```python
from build123d import *

# Parameters (mm, degrees)
SKETCH1_W           = 25
SKETCH1_H           = 60
BOSS_EXTRUDE1_DEPTH = 30
SKETCH2_W           = 60
SKETCH2_H           = 8.623813306
BOSS_EXTRUDE2_DEPTH = 20
SKETCH3_R           = 4
CUT_EXTRUDE1_DEPTH  = 9.623813306
CUT_EXTRUDE2_DEPTH  = 20
BOSS_EXTRUDE3_DEPTH = 1


with BuildPart() as part:
    # Sketch1 → Boss-Extrude1 (new body)
    with BuildSketch(Plane(origin=(0, 0, 0), x_dir=(1, 0, 0), z_dir=(0, 1, 0))):
        Rectangle(SKETCH1_W, SKETCH1_H)
    extrude(amount=BOSS_EXTRUDE1_DEPTH)

    # Sketch2 → Boss-Extrude2 (add)
    with BuildSketch(Plane.ZY.offset(12.5)):
        with Locations((0, 4.311906653)):
            Rectangle(SKETCH2_W, SKETCH2_H)
    extrude(amount=BOSS_EXTRUDE2_DEPTH)

    # Sketch3 → Cut-Extrude1 (cut, through all)
    with BuildSketch(Plane(origin=(0, 8.623813306, 0), x_dir=(1, 0, 0), z_dir=(0, 1, 0))):
        with Locations(Location((-24.5, 20, 0), (0, 0, 270))):  # turned: the seam where the file's is
            Circle(SKETCH3_R)
        with Locations(Location((-24.5, -20, 0), (0, 0, 270))):  # turned: the seam where the file's is
            Circle(SKETCH3_R)
    extrude(amount=-CUT_EXTRUDE1_DEPTH, mode=Mode.SUBTRACT)

    # Sketch4 → Cut-Extrude2 (cut)
    with BuildSketch(Plane(origin=(12.5, 0, 0), x_dir=(0, 0, -1), z_dir=(1, 0, 0))):
        Polygon((12.414671802, 26.015265685), (25.398981518, 10.541167934), (17.585328198, 3.984734315), (4.601018482, 19.458832066), align=None)
    extrude(amount=-CUT_EXTRUDE2_DEPTH, mode=Mode.SUBTRACT)

    # Sketch5 → Boss-Extrude3 (add)
    with BuildSketch(Plane(origin=(0, 30, 0), x_dir=(1, 0, 0), z_dir=(0, 1, 0))):
        with BuildLine():
            Line((7.692307692, 10), (7.692307692, -10))
            Line((7.692307692, -10), (-0.985576923, -10))
            add(Edge.make_bspline(
                [(-0.985576923, -10), (-1.189915508, -9.998406517), (-1.585388921, -9.995322517), (-2.158891161, -9.97328499), (-2.692933181, -9.926466249), (-3.190880742, -9.87417544), (-3.651881782, -9.796967041), (-4.076156001, -9.706387661), (-4.462076213, -9.599333368), (-4.812578849, -9.472790754), (-5.13779529, -9.329673653), (-5.439160579, -9.1529927), (-5.729614752, -8.959721513), (-5.997579665, -8.730765608), (-6.255124362, -8.484777239), (-6.491466209, -8.20944831), (-6.713599726, -7.911670049), (-6.98368474, -7.480457665), (-7.26734754, -6.902448182), (-7.511671117, -6.168093018), (-7.667028651, -5.399134972), (-7.683798939, -4.873873893), (-7.692307692, -4.607371795)],
                knots=[0, 0, 0, 0, 1.242075696, 2.40389213, 3.487198984, 4.500157661, 5.446319301, 6.326791195, 7.136300648, 7.878370406, 8.590488565, 9.292260633, 9.999224673, 10.708050372, 11.431369221, 12.162165018, 12.910600795, 13.687589445, 15.252257874, 16.810406251, 18.381693487, 20, 20, 20, 20], degree=3))
            add(Edge.make_bspline(
                [(-7.692307692, -4.607371795), (-7.688394011, -4.436288612), (-7.680664221, -4.098387595), (-7.621454116, -3.601582104), (-7.51431592, -3.126906532), (-7.376939813, -2.670193942), (-7.1888858, -2.237951011), (-6.971132957, -1.821215885), (-6.700987613, -1.431932834), (-6.399355855, -1.057091635), (-6.048612719, -0.71360816), (-5.658467411, -0.39614679), (-5.217190586, -0.123711561), (-4.739255324, 0.129469087), (-4.212344466, 0.337396306), (-3.644404331, 0.520482963), (-3.031039376, 0.661647942), (-2.605906991, 0.732754289), (-2.387820513, 0.769230769)],
                knots=[0, 0, 0, 0, 0.982645791, 1.940792824, 2.867691729, 3.775150443, 4.675643875, 5.571354211, 6.471357401, 7.392684514, 8.331098131, 9.285922955, 10.275520706, 11.304845665, 12.388884831, 13.524255008, 14.729980297, 16, 16, 16, 16], degree=3))
            add(Edge.make_bspline(
                [(-2.387820513, 0.769230769), (-2.549345996, 0.849743746), (-2.855664626, 1.002429402), (-3.272498706, 1.255059029), (-3.637663897, 1.492888205), (-3.845092801, 1.671226556), (-3.942307692, 1.754807692)],
                knots=[0, 0, 0, 0, 1.172551213, 2.223638478, 3.167479604, 4, 4, 4, 4], degree=3))
            add(Edge.make_bspline(
                [(-3.942307692, 1.754807692), (-4.131560958, 1.939760877), (-4.519688241, 2.319069404), (-5.049338611, 2.971134565), (-5.573421338, 3.688219618), (-5.888069662, 4.2107727), (-6.049679487, 4.479166667)],
                knots=[0, 0, 0, 0, 0.918170575, 1.883016652, 2.912673989, 4, 4, 4, 4], degree=3))
            Line((-6.049679487, 4.479166667), (-9.330929487, 10))
            Line((-9.330929487, 10), (-6.09775641, 10))
            Line((-6.09775641, 10), (-3.605769231, 5.77724359))
            add(Edge.make_bspline(
                [(-3.605769231, 5.77724359), (-3.516164402, 5.629086783), (-3.342524957, 5.34198322), (-3.091798881, 4.922621923), (-2.845639404, 4.536751784), (-2.618440056, 4.172360633), (-2.395792195, 3.839058208), (-2.196203285, 3.524230537), (-1.99576396, 3.245712753), (-1.765615132, 2.91110533), (-1.484546035, 2.549334189), (-1.156558274, 2.177690005), (-0.854995349, 1.869836465), (-0.473923576, 1.576103263), (-8.0808e-05, 1.307161834), (0.399436219, 1.179583217), (0.592948718, 1.117788462)],
                knots=[0, 0, 0, 0, 1.130591283, 2.190900266, 3.190104209, 4.119071823, 4.994606968, 5.807262858, 6.55236009, 7.234593472, 8.459046683, 9.540234366, 10.471327768, 11.266723835, 12.676093724, 14, 14, 14, 14], degree=3))
            add(Edge.make_bspline(
                [(0.592948718, 1.117788462), (0.674242958, 1.103128347), (0.859840146, 1.069658866), (1.174983707, 1.047799895), (1.556818794, 1.024599522), (1.833541189, 1.025275503), (1.983173077, 1.025641026)],
                knots=[0, 0, 0, 0, 0.709978628, 1.620902492, 2.713552433, 4, 4, 4, 4], degree=3))
            Line((1.983173077, 1.025641026), (4.871794872, 1.025641026))
            Line((4.871794872, 1.025641026), (4.871794872, 10))
            Line((4.871794872, 10), (7.692307692, 10))
        make_face()
        with BuildLine():
            Line((4.871794872, -1.282051282), (-0.484775641, -1.282051282))
            add(Edge.make_bspline(
                [(-0.484775641, -1.282051282), (-0.753386517, -1.286217416), (-1.255529355, -1.294005613), (-1.957518176, -1.361528247), (-2.558000395, -1.467075801), (-3.064646298, -1.627384754), (-3.490432782, -1.842070076), (-3.859462924, -2.104609449), (-4.169752828, -2.430321342), (-4.424939479, -2.80379836), (-4.624425797, -3.210810832), (-4.763816724, -3.641583566), (-4.857398907, -4.087856282), (-4.866967535, -4.393220511), (-4.871794872, -4.547275641)],
                knots=[0, 0, 0, 0, 1.546056516, 2.890207646, 4.055830773, 5.050253158, 5.937355789, 6.790906573, 7.644595853, 8.512568064, 9.38593768, 10.244184789, 11.114197691, 12, 12, 12, 12], degree=3))
            add(Edge.make_bspline(
                [(-4.871794872, -4.547275641), (-4.868088958, -4.659544766), (-4.86083016, -4.879447), (-4.822372143, -5.202097101), (-4.749202425, -5.50786025), (-4.648165007, -5.798940542), (-4.520236894, -6.075969951), (-4.363033481, -6.337858904), (-4.177365929, -6.583269781), (-3.964383478, -6.81341075), (-3.719926868, -7.02284832), (-3.440676061, -7.203538998), (-3.128860999, -7.357089463), (-2.784111469, -7.478956731), (-2.407515729, -7.576430897), (-1.996929252, -7.641277267), (-1.554229928, -7.688199899), (-1.24746496, -7.690912847), (-1.08974359, -7.692307692)],
                knots=[0, 0, 0, 0, 0.965235723, 1.89061323, 2.787065514, 3.661873922, 4.534873316, 5.404925039, 6.281839248, 7.175200054, 8.095223355, 9.040740021, 10.02630299, 11.075573487, 12.177989335, 13.364883635, 14.645170704, 16, 16, 16, 16], degree=3))
            Line((-1.08974359, -7.692307692), (4.871794872, -7.692307692))
            Line((4.871794872, -7.692307692), (4.871794872, -1.282051282))
        make_face(mode=Mode.SUBTRACT)
    extrude(amount=BOSS_EXTRUDE3_DEPTH)


solid = part.part
```
For this review, take the finished solid that the model builds, in its own axes (mm). A direction names the side the tool comes from. Round coordinates to 2 decimals unless told otherwise and drop trailing zeros. Write each loop counter-clockwise with the first axis right and the second up, starting at its lowest first coordinate (ties: lowest second). Pieces come first, ordered by that corner, then holes. Notation, with made-up numbers: M -8.5,-37 L -3.5,-37 A22 ccw -3.5,-4 Z; hole C 46.25,82.25 d10. An arc over 180 degrees is marked long. One line per item, written item: value. Start each with the question number.
(1) We need section D-D (z = 11). Give the boundary of the cut face in (x, y), and give its area (3 significant figures).
(2) We need section A-A (z = 20). Give the boundary of the cut face in (x, y).
(3) We need section C-C (x = 3). Give the boundary of the cut face in (y, z).
(4) Insertion check: pin 1 (0.8 mm diameter, centred on x = 3.5, y = 30.5, fed in from +Z); pin 2 (0.8 mm diameter, centred on y = 30.5, z = -3.5, fed in from +X); pin 3 (1.1 mm diameter, centred on y = 30.5, z = 3.5, fed in from -X). Each pin has a flat end and moves straight along its axis. Give the tip position at first contact, or say it passes through.
(5) We need section B-B (x = -24.5). Give the boundary of the cut face in (y, z), and give its area (3 significant figures).
(6) The part is to be moulded in two halves that separate along Y. For faces 1 (the flat face through (2.64, 7.31, -21.55)), 2 (the flat face through (-32.5, 4, 0)), 3 (the flat face through (-10, 0, 0)), say which applies: released by +Y, released by -Y, zero draft, split by the parting line, or undercut.
(7) Machinability: for faces 4 (the flat face through (-7.5, 15, -15)), 5 (the flat face through (0, 30, 4)), 6 (the flat face through (-4.87, 30.49, -7.92)), which of the approach directions +Z, -Z, +X, -X, +Y, -Y give a long, thin tool a straight path to every point of the face, cutting with its end or side? Answer none if there is none.
(8) Wall thickness on line 1 (Z direction, x = -24, y = 2); line 2 (X direction, y = 4, z = -20); line 3 (Y direction, x = -14, z = 10.5): over which ranges is each line inside the solid? List them lowest first.
Result:
1. outline: M -32.5,0 L 12.5,0 L 12.5,30 L -12.5,30 L -12.5,8.62 L -32.5,8.62 Z
1. area: 922 mm²
2. outline: M -32.5,0 L -28.5,0 L -28.5,8.62 L -32.5,8.62 Z; M -20.5,0 L 12.5,0 L 12.5,30 L -12.5,30 L -12.5,8.62 L -20.5,8.62 Z
3. outline: M 0,-30 L 30,-30 L 30,-1.03 L 31,-1.03 L 31,1.28 L 30,1.28 L 30,7.69 L 31,7.69 L 31,10 L 30,10 L 30,30 L 0,30 Z; hole M 3.98,-17.59 L 10.54,-25.4 L 26.02,-12.41 L 19.46,-4.6 Z
4. pin 1: z = 10
4. pin 2: x = 7.69
4. pin 3: x = -12.5
5. outline: M 0,-30 L 8.62,-30 L 8.62,-24 L 0,-24 Z; M 0,-16 L 8.62,-16 L 8.62,16 L 0,16 Z; M 0,24 L 8.62,24 L 8.62,30 L 0,30 Z
5. area: 379 mm²
6. face 1: undercut
6. face 2: zero draft
6. face 3: released by -Y
7. face 4: +X
7. face 5: +Y
7. face 6: -Z, +Y
8. line 1: -30 to -23.97, -16.03 to 16.03, 23.97 to 30
8. line 2: -32.5 to -28.5, -20.5 to 12.5
8. line 3: 0 to 8.62
